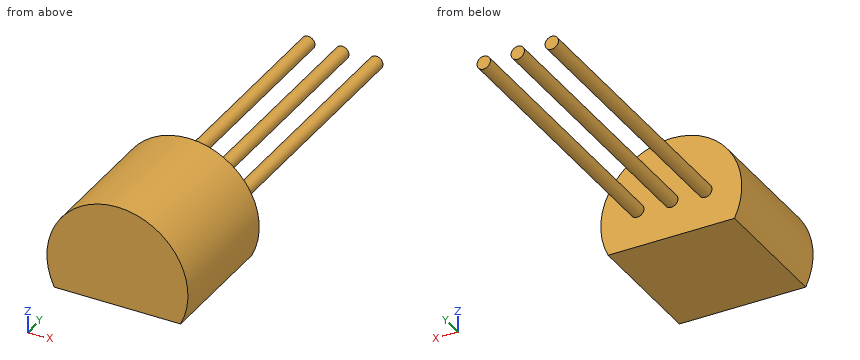
from build123d import *

# Parameters (mm, degrees)
BOSS_EXTRUDE1_DEPTH = 5.33
SKETCH2_R           = 0.275
BOSS_EXTRUDE2_DEPTH = 11.48431719


with BuildPart() as part:
    # Sketch1 → Boss-Extrude1 (new body)
    with BuildSketch(Plane(origin=(0, 0, 0), x_dir=(1, 0, 0), z_dir=(0, 1, 0))):
        with BuildLine():
            Line((-2.6, 0), (2.6, 0))
            ThreePointArc((2.6, 0), (0, -4.19), (-2.6, 0))
        make_face()
    extrude(amount=BOSS_EXTRUDE1_DEPTH)

    # Sketch2 → Boss-Extrude2 (add)
    with BuildSketch(Plane(origin=(0, 5.33, 0), x_dir=(1, 0, 0), z_dir=(0, 1, 0))):
        with Locations((0, -1.53)):
            Circle(SKETCH2_R)
        with Locations((-1.4, -1.53)):
            Circle(SKETCH2_R)
        with Locations((1.4, -1.53)):
            Circle(SKETCH2_R)
    extrude(amount=BOSS_EXTRUDE2_DEPTH)


solid = part.part
Verification items for the finished model (mm, model axes). Round coordinates to 2 decimals unless told otherwise and drop trailing zeros. Loops run counter-clockwise (first coordinate to the right, second up) from the corner with the lowest first, then second, coordinate; pieces in that order, holes last. Notation, with made-up numbers: (-22.5, 20) - (-7.5, 20) arc R12 ccw to (-7.5, 42) - close; hole circle Ø4 at (52, 86). An arc over 180 degrees is marked (long way). Write item = value, one per line.
Q1. Depth check by flat-ended pin: pin 1 (1.3 mm diameter, centred on x = 1, z = 2.5, fed in from +Y). Enter the tip coordinate at first touch or a pass-through.
Here are the results:
pin_1 = 5.33
Q2. Sectioned sample at C-C on z = 1.53. Record the boundary of the cut face in (x, y) (3 decimals).
Here are the results:
outline = (-2.892, 0) - (2.892, 0) - (2.892, 5.33) - (1.675, 5.33) - (1.675, 16.814) - (1.125, 16.814) - (1.125, 5.33) - (0.275, 5.33) - (0.275, 16.814) - (-0.275, 16.814) - (-0.275, 5.33) - (-1.125, 5.33) - (-1.125, 16.814) - (-1.675, 16.814) - (-1.675, 5.33) - (-2.892, 5.33) - close
Q3. Sectioned sample at D-D on x = 1.4. Record the boundary of the cut face in (y, z) (3 decimals).
Here are the results:
outline = (0, 0) - (5.33, 0) - (5.33, 1.255) - (16.814, 1.255) - (16.814, 1.805) - (5.33, 1.805) - (5.33, 3.83) - (0, 3.83) - close
Q4. Sectioned sample at B-B on x = 0. Record the boundary of the cut face in (y, z) (3 decimals).
Here are the results:
outline = (0, 0) - (5.33, 0) - (5.33, 1.255) - (16.814, 1.255) - (16.814, 1.805) - (5.33, 1.805) - (5.33, 4.19) - (0, 4.19) - close
Q5. Material ranges on L1, parallel to Y at x = 1.05, z = 3.4; L2, parallel to Z at x = -0.05, y = 13.75; L3, parallel to Z at x = -1.15, y = 3.25, recorded low to high.
Here are the results:
L1 = 0 to 5.33
L2 = 1.26 to 1.8
L3 = 0 to 3.95
Q6. Sectioned sample at A-A on y = 10. Record the boundary of the cut face in (x, z) (3 decimals), plus the area to 3 significant figures.
Here are the results:
outline = circle Ø0.55 at (-1.4, 1.53); circle Ø0.55 at (0, 1.53); circle Ø0.55 at (1.4, 1.53)
area = 0.713 mm^2
